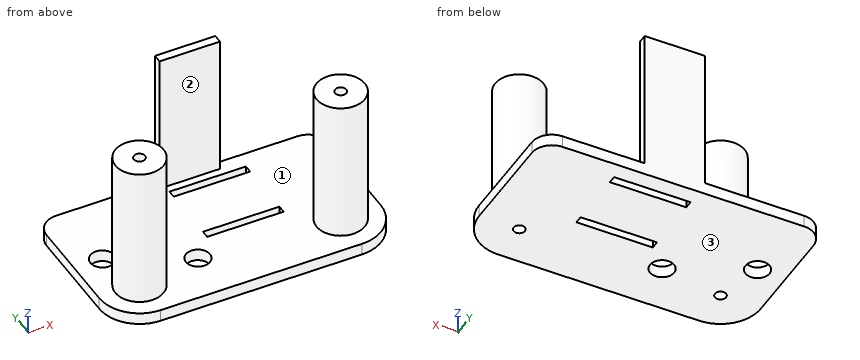
from build123d import *

# Parameters (mm, degrees)
F0_R     = 6
F0_R_2   = 1.4
F1_DEPTH = 39
F0_W     = 15
F0_H     = 2.2
F0_R_3   = 3
F0_W_2   = 19
F0_H_2   = 2
F2_DEPTH = 3


with BuildPart() as f1:
    # F0 (on Top) → F1 (new body)
    with BuildSketch(Plane.XY):
        with Locations((25, -10)):
            Circle(F0_R)
        with Locations((25, -10)):
            Circle(F0_R_2, mode=Mode.SUBTRACT)
    extrude(amount=F1_DEPTH)



with BuildPart() as f1b:
    # F0 (on Top) → F1, piece 2 (new body)
    with BuildSketch(Plane.XY):
        with Locations((-25, -10)):
            Circle(F0_R)
        with Locations((-25, -10)):
            Circle(F0_R_2, mode=Mode.SUBTRACT)
    extrude(amount=F1_DEPTH)


with BuildPart() as f1c:
    # F0 (on Top) → F1, piece 3 (new body)
    with BuildSketch(Plane.XY):
        with Locations((2.0735195652, 18.9)):
            Rectangle(F0_W, F0_H)
    extrude(amount=F1_DEPTH)


with BuildPart() as f1_1:
    add(f1.part)

    add(f1b.part)  # F2 merges F1b

    add(f1c.part)  # F2 merges F1c
    # F0 (on Top) → F2 (join)
    with BuildSketch(Plane.XY):
        with BuildLine():
            ThreePointArc((35, 15), (33.5355339059, 18.5355339059), (30, 20))
            Line((30, 20), (9.5735195652, 20))
            Line((9.5735195652, 20), (9.5735195652, 17.8))
            Line((9.5735195652, 17.8), (-5.4264804348, 17.8))
            Line((-5.4264804348, 17.8), (-5.4264804348, 20))
            Line((-5.4264804348, 20), (-30, 20))
            ThreePointArc((-30, 20), (-33.5355339059, 18.5355339059), (-35, 15))
            Line((-35, 15), (-35, -10))
            ThreePointArc((-35, -10), (-32.0710678119, -17.0710678119), (-25, -20))
            Line((-25, -20), (25, -20))
            ThreePointArc((25, -20), (32.0710678119, -17.0710678119), (35, -10))
            Line((35, -10), (35, 15))
        make_face()
        with Locations((-25, -10)):
            Circle(F0_R, mode=Mode.SUBTRACT)
        with Locations((-9.2434035614, -7.6480722055)):
            Circle(F0_R_3, mode=Mode.SUBTRACT)
        with Locations((5.526580222, -1)):
            Rectangle(F0_W_2, F0_H_2, mode=Mode.SUBTRACT)
        with Locations((25, -10)):
            Circle(F0_R, mode=Mode.SUBTRACT)
        with Locations((-28, 1.8378978129)):
            Circle(F0_R_3, mode=Mode.SUBTRACT)
        with Locations((5.526580222, 14.8842966408)):
            Rectangle(F0_W_2, F0_H_2, mode=Mode.SUBTRACT)
        with Locations((2.0735195652, 18.9)):
            Rectangle(F0_W, F0_H)
    extrude(amount=F2_DEPTH)


solid = f1_1.part
Design review of the part built by this model. Coordinates are the model's own, in mm. Face numbers are marked on the shaded views. A direction names the side the tool comes from. Coordinates: 2 decimals unless noted, no trailing zeros. Loops run counter-clockwise (first coordinate to the right, second up) from the corner with the lowest first, then second, coordinate; pieces in that order, holes last.
Item 1: Add section B-B (z = 36.5). Write out the cut boundary in (x, y), and give its area (3 significant figures).
Completed:
outline: circle Ø12 at (-25, -10); (-5.43, 17.8) - (9.57, 17.8) - (9.57, 20) - (-5.43, 20) - close; circle Ø12 at (25, -10); hole circle Ø2.8 at (-25, -10); hole circle Ø2.8 at (25, -10)
area: 247 mm2
Item 2: Wall thickness on L1, parallel to X at y = -9, z = 29.5; L2, parallel to Z at x = 13, y = -4; L3, parallel to Y at x = -25.5, z = 24: over which ranges is each line inside the solid? List them lowest first.
Completed:
L1: x = -30.92 to -25.98, -24.02 to -19.08, 19.08 to 24.02, 25.98 to 30.92
L2: z = 0 to 3
L3: y = -15.98 to -11.31, -8.69 to -4.02
Item 3: Clearance check with flat-ended pins moving along their axes: pin 1 (5 mm diameter, centred on x = -6, z = 12.5, fed in from +Y); pin 2 (10 mm diameter, centred on x = -4, z = 30.5, fed in from -Y); pin 3 (12 mm diameter, centred on x = 4, y = -9.5, fed in from +Z); pin 4 (2.5 mm diameter, centred on y = 18.5, z = 14.5, fed in from +X). State where each tip first meets the part, or that it passes through.
Completed:
pin 1: stops at y = 20
pin 2: stops at y = 17.8
pin 3: stops at z = 3
pin 4: stops at x = 9.57
Item 4: Add section C-C (x = -28). Write out the cut boundary in (y, z), and give its area (3 significant figures).
Completed:
outline: (-19.54, 0) - (-1.16, 0) - (-1.16, 3) - (-4.8, 3) - (-4.8, 39) - (-15.2, 39) - (-15.2, 3) - (-19.54, 3) - close; (4.84, 0) - (20, 0) - (20, 3) - (4.84, 3) - close
area: 475 mm2
Item 5: Add section D-D (y = -14.5). Write out the cut boundary in (x, z).
Completed:
outline: (-33.93, 0) - (33.93, 0) - (33.93, 3) - (28.97, 3) - (28.97, 39) - (21.03, 39) - (21.03, 3) - (-21.03, 3) - (-21.03, 39) - (-28.97, 39) - (-28.97, 3) - (-33.93, 3) - close
Item 6: For the marked faces 1, 2 and 3, list the 3-axis set-ups (+Z, -Z, +X, -X, +Y, -Y) from which the entire face can be reached by the end or side of a thin tool; tool diameter is ignored.
Completed:
face 1: +Z
face 2: +Z, +X, -X, -Y
face 3: -Z, +X, -X, +Y, -Y
Item 7: Add section A-A (x = 3). Write out the cut boundary in (y, z), and give its area (3 significant figures).
Completed:
outline: (-20, 0) - (-2, 0) - (-2, 3) - (-20, 3) - close; (0, 0) - (13.88, 0) - (13.88, 3) - (0, 3) - close; (15.88, 0) - (20, 0) - (20, 39) - (17.8, 39) - (17.8, 3) - (15.88, 3) - close
area: 187 mm2
